The listing builds one solid part. Answer for the finished solid, in the listing's coordinates (mm). A direction names the side the tool comes from. Give positions to 0.01 mm unless a question says otherwise; leave off trailing zeros. Loops run counter-clockwise (first coordinate to the right, second up) from the corner with the lowest first, then second, coordinate; pieces in that order, holes last. Notation, with made-up numbers: (0.25, -7) - (33.25, -7) arc R15 cw to (33.25, 17) - close; hole circle Ø11 at (71.5, 62.25). An arc over 180 degrees is marked (long way). Answer in a Markdown table with one row per item. Add a question column.
```python
from build123d import *

# Parameters (mm, degrees)
F1_DEPTH = 20.82483
F2_R     = 11.219442
F3_DEPTH = 25.4
F4_R     = 6.603973
F5_DEPTH = 39.32976


with BuildPart() as f1:
    # F0 (on Top) → F1 (new body)
    with BuildSketch(Plane.XY):
        with BuildLine():
            Line((0, 0), (-9.817178, 0))
            ThreePointArc((-9.817178, 0), (-13.732727, 14.634683), (-25.851902, 23.724847))
            Line((-25.851902, 23.724847), (-25.851902, 36.487177))
            Line((-25.851902, 36.487177), (-43.195583, 36.487177))
            Line((-43.195583, 36.487177), (-43.195583, 23.724847))
            ThreePointArc((-43.195583, 23.724847), (-54.642663, 14.114905), (-59.557546, 0))
            Line((-59.557546, 0), (-69.374725, 0))
            Line((-69.374725, 0), (-69.374725, -7.690122))
            Line((-69.374725, -7.690122), (0, -7.690122))
            Line((0, -7.690122), (0, 0))
        make_face()
    extrude(amount=F1_DEPTH)

    # F2 (on Top) → F3 (cut)
    with BuildSketch(Plane.XY):
        with Locations((-33.670925, 8.802438)):
            Circle(F2_R)
    extrude(amount=F3_DEPTH, mode=Mode.SUBTRACT)

    # F4 (on Front) → F5 (cut)
    with BuildSketch(Plane.XZ):
        with Locations((-34.637902, 10.000476)):
            Circle(F4_R)
    extrude(amount=-F5_DEPTH, mode=Mode.SUBTRACT)


solid = f1.part
```
(1) The mould has two halves that part along Z. Classify faces 1 (the face through (-43.196, 30, 10)), 2 (the face through (-41.235, 26.649, 10.291)), 3 (the face through (-27, 20, 20.825)), 4 (the face through (-27, 20, 0)): pulls with the +Z half, pulls with the -Z half, needs draft (parallel to the pull), parting line crosses it, or undercut.
(2) Given pin 1 Ø3 at (x, z) = (-55.5, 3.5) entering from +Y; pin 2 Ø20 at (x, y) = (-33.67, 8.8) entering from +Z; pin 3 Ø10 at (y, z) = (30.5, 14) entering from +X; pin 4 Ø10 at (y, z) = (22, 11) entering from -X, each flat-ended and moving along its own axis, determine where each tip first touches the part or whether it passes through.
(3) A tool of negligible diameter and unlimited length cuts with its end or side. For faces 5 (the face through (-64, 0, 10)), 6 (the face through (-25.852, 30, 10)), 7 (the face through (-35, -7.69, 10)), from which of +Z, -Z, +X, -X, +Y, -Y can it reach the whole face along a straight path? Write none if from no direction.
(4) A cutting plane is placed at D-D on y = 27. Determine the outline of the cut face in (x, z), plus the area to 3 significant figures.
(5) A cutting plane is placed at C-C on z = 19.75. Determine the outline of the cut face in (x, y).
(6) A cutting plane is placed at A-A on y = 11. Determine the outline of the cut face in (x, z).
(7) A cutting plane is placed at B-B on x = -38. Determine the outline of the cut face in (y, z).
(8) Find the intervals of material crossed by line 1 along X through (y, z) = (12.5, 1.5); line 2 along Y through (x, z) = (-4, 4); line 3 along X through (y, z) = (29, 12), in increasing order. Write a range as [from, to].
Evaluation:
| question | item | result |
|---|---|---|
| 1 | face 1 | needs draft |
| 1 | face 2 | undercut |
| 1 | face 3 | pulls with the +Z half |
| 1 | face 4 | pulls with the -Z half |
| 2 | pin 1 | stops at y = 15.01 |
| 2 | pin 2 | passes through |
| 2 | pin 3 | stops at x = -25.85 |
| 2 | pin 4 | stops at x = -52.36 |
| 3 | face 5 | +Z, -Z, -X, +Y |
| 3 | face 6 | +Z, -Z, +X, +Y |
| 3 | face 7 | +Z, -Z, +X, -X, -Y |
| 4 | outline | (-43.2, 0) - (-25.85, 0) - (-25.85, 20.82) - (-43.2, 20.82) - close; hole circle Ø13.21 at (-34.64, 10) |
| 4 | area | 224 mm² |
| 5 | outline | (-69.37, -7.69) - (0, -7.69) - (0, 0) - (-9.82, 0) arc R23.18 ccw to (-25.85, 23.72) - (-25.85, 36.49) - (-43.2, 36.49) - (-43.2, 23.72) arc R28.15 ccw to (-59.56, 0) - (-69.37, 0) - close; hole circle Ø22.44 at (-33.67, 8.8) |
| 6 | outline | (-56.51, 0) - (-44.67, 0) - (-44.67, 20.82) - (-56.51, 20.82) - close; (-22.67, 0) - (-11.73, 0) - (-11.73, 20.82) - (-22.67, 20.82) - close |
| 7 | outline | (-7.69, 0) - (-1.55, 0) - (-1.55, 20.82) - (-7.69, 20.82) - close; (19.15, 0) - (36.49, 0) - (36.49, 4.32) - (19.15, 4.32) - close; (19.15, 15.68) - (36.49, 15.68) - (36.49, 20.82) - (19.15, 20.82) - close |
| 8 | line 1 | x = [-55.68, -44.26], [-23.08, -12.45] |
| 8 | line 2 | y = [-7.69, 0] |
| 8 | line 3 | x = [-43.2, -40.93], [-28.34, -25.85] |
